from build123d import *


with BuildPart() as part:
    # Esquisse1 → R_volution1 (revolve)
    with BuildSketch(Plane(origin=(0, 0, 0), x_dir=(0, 0, -1), z_dir=(1, 0, 0)), mode=Mode.PRIVATE) as r_volution1_sk:
        Polygon((-1.7, 10), (-2, 9.7), (-2, 7.8), (-1.7, 7.5), (3.2, 7.5), (3.5, 7.8), (3.5, 9.7), (3.2, 10), align=None)
    revolve(r_volution1_sk.sketch.rotate(Axis((0, 0, 10.3632), (0, 0, -1)), 90), axis=Axis((0, 0, 10.3632), (0, 0, -1)))


solid = part.part
Build history of the part. All positions in model axes, mm. Give positions to 0.01 mm unless a question says otherwise; leave off trailing zeros. Loops run counter-clockwise (first coordinate to the right, second up) from the corner with the lowest first, then second, coordinate; pieces in that order, holes last. Notation, with made-up numbers: (65.25, 60) - (120.25, 60) arc R13 ccw to (120.25, 77) - close; hole circle Ø11 at (-19, 10). An arc over 180 degrees is marked (long way). Write item = value, one per line. Start each with the question number.
1) Band-saw the part on C-C on z = -0.35. Give the cut face in (x, y), plus the area to 3 significant figures.
2) Pull direction X, two halves, no side cores. Call faces 1 (the cylindrical face through (4.032, -6.324, -0.784)), 2 (the flat face through (7, -4, -3.5)), 3 (the cylindrical face through (-10, 0, -1)): +X half, -X half, draft (parallel to the pull), parting line (faces both ways), or undercut.
3) Probe probe 1 along Y at (x, z) = (0, -0.8); probe 2 along X at (y, z) = (3.5, -2.6); probe 3 along X at (y, z) = (-6, 0.15). List the from-to ranges inside material, lowest first. Write a range as from..to.
4) Drop a flat-ended pin along its axis: pin 1 Ø1 at (y, z) = (-1.5, -3) entering from -X. Give the stop position or say it passes through.
5) Band-saw the part on A-A on x = 0. Give the cut face in (y, z).
Final values:
q1.outline = circle Ø20 at (0, 0); hole circle Ø15 at (0, 0)
q1.area = 137 mm²
q2.face_1 = undercut
q2.face_2 = draft
q2.face_3 = parting line
q3.probe_1 = -10..-7.5, 7.5..10
q3.probe_2 = -9.37..-6.63, 6.63..9.37
q3.probe_3 = -8..-4.5, 4.5..8
q4.pin_1 = -9.95
q5.outline = (-10, -3.2) - (-9.7, -3.5) - (-7.8, -3.5) - (-7.5, -3.2) - (-7.5, 1.7) - (-7.8, 2) - (-9.7, 2) - (-10, 1.7) - close; (7.5, -3.2) - (7.8, -3.5) - (9.7, -3.5) - (10, -3.2) - (10, 1.7) - (9.7, 2) - (7.8, 2) - (7.5, 1.7) - close
